Here's how the part is built. I have some questions about the finished solid (model axes, mm). A direction names the side the tool comes from. Round coordinates to 2 decimals unless told otherwise and drop trailing zeros. Loops run counter-clockwise (first coordinate to the right, second up) from the corner with the lowest first, then second, coordinate; pieces in that order, holes last. Notation, with made-up numbers: M 34,15 L 64,15 A19 ccw 64,33 Z; hole C 75,-32 d7. An arc over 180 degrees is marked long. Use a Markdown table: item, result.
from build123d import *

# Parameters (mm, degrees)
SKETCH2_W                = 3.0000000000000036
SKETCH2_H                = 3.9999999999999982
BOSS_EXTRUDE2_DEPTH      = 100
BOSS_EXTRUDE3_DEPTH      = 30
BOSS_EXTRUDE3_DEPTH_BACK = 105
FILLET5_R                = 10
FILLET6_R                = 5
FILLET7_R                = 2
FILLET8_R                = 1


with BuildPart() as part:
    # Sketch2 → Boss-Extrude2 (new body)
    with BuildSketch(Plane(origin=(0, 0, 0), x_dir=(0, 0, -1), z_dir=(1, 0, 0))):
        Polygon((8.660254037844407, 18.999999999999996), (24.660254037844407, 19), (27.660254037844407, 19), (27.660254037844407, 23), (8.660254037844407, 22.999999999999996), align=None)
        with Locations((26.160254037844403, 17)):
            Rectangle(SKETCH2_W, SKETCH2_H)
        Polygon((24.660254037844407, 15), (18.66025403784441, 15), (16.3508529610859, 10.999999999999996), (27.66025403784441, 11), (27.660254037844407, 15), align=None)
        Polygon((18.66025403784441, 15), (8.660254037844407, 15), (8.660254037844409, 11), (16.3508529610859, 11), align=None)
        with BuildLine():
            Line((8.660254037844407, 15.000000000000002), (0, 0))
            Line((0, 0), (3.2679491924311206, 1.4e-16))
            Line((3.2679491924311206, -8.2e-16), (6.165063509461155, 5.017949192431213))
            ThreePointArc((6.165063509461059, 5.017949192431232), (7.962900689456138, 8.449244298165432), (10.964101615137764, 6))
            ThreePointArc((10.964101615137764, 5.999999999999999), (10.334608934582356, 4.341325116876664), (8.763139720814397, 3.5179491924311193))
            Line((8.763139720814408, 3.5179491924311046), (6.732050807568877, 0))
            Line((6.732050807568877, 2.8e-16), (10.000000000000004, 4.1e-16))
            Line((10.000000000000004, -1.78e-15), (16.3508529610859, 10.999999999999996))
            Line((16.3508529610859, 11), (8.660254037844409, 11))
            Line((8.660254037844409, 11), (8.660254037844407, 15))
        make_face()
    extrude(amount=BOSS_EXTRUDE2_DEPTH)

    # Sketch3 → Boss-Extrude3 (add, two sides: drawn at the far end of the back side and taken through both)
    with BuildSketch(Plane(origin=(100, 0, 0), x_dir=(0, 0, -1), z_dir=(1, 0, 0)).offset(-BOSS_EXTRUDE3_DEPTH_BACK)):
        with BuildLine():
            Line((8.66025403784439, 15.000000000000005), (0, 0))
            Line((0, 0), (3.2679491924311215, 2.8e-16))
            Line((3.267949192431121, 0), (6.1650635094611035, 5.017949192431125))
            ThreePointArc((6.165063509461104, 5.017949192431125), (7.962900689456081, 8.449244298165421), (10.964101615137764, 6))
            ThreePointArc((10.964101615137764, 5.999999999999999), (10.334608934582363, 4.341325116876672), (8.763139720814419, 3.517949192431122))
            Line((8.763139720814419, 3.517949192431122), (6.732050807568878, 3.6e-16))
            Line((6.732050807568878, 3.6e-16), (10.000000000000002, 8.7e-16))
            Line((10.000000000000004, 0), (18.66025403784441, 15.000000000000009))
            Line((18.66025403784441, 15.000000000000009), (8.66025403784439, 15.000000000000005))
        make_face()
    extrude(amount=BOSS_EXTRUDE3_DEPTH + BOSS_EXTRUDE3_DEPTH_BACK)

    # Fillet5
    fillet5_edges = [part.edges().sort_by_distance(p)[0] for p in [
        (50, 10.999999999999998, -16.3508529610859),
    ]]
    fillet(fillet5_edges, radius=FILLET5_R)

    # Fillet6
    fillet6_edges = [part.edges().sort_by_distance(p)[0] for p in [
        (0, 10.500000000000007, -16.062177826491087),
        (100, 10.500000000000007, -16.062177826491087),
    ]]
    fillet(fillet6_edges, radius=FILLET6_R - 0.0001)  # a hair under: the kernel refuses the full size

    # Fillet7
    fillet7_edges = [part.edges().sort_by_distance(p)[0] for p in [
        (50, 23, -27.660254037844407),
        (50, 11, -27.66025403784441),
    ]]
    fillet(fillet7_edges, radius=FILLET7_R)

    # Fillet8
    fillet8_edges = [part.edges().sort_by_distance(p)[0] for p in [
        (62.5, 4.3e-16, -10.000000000000004),
        (62.5, 0, 0),
    ]]
    fillet(fillet8_edges, radius=FILLET8_R)


solid = part.part
1. I need wall thicknesses on probe 1 along Y at (x, z) = (2, -10.25); probe 2 along X at (y, z) = (12.5, -26); probe 3 along Y at (x, z) = (48, -16.5). Which ranges of each line are inside material? Lowest first, please. Write a range as from..to.
Answer sheet:
| item | result |
|---|---|
| probe 1 | 0.44..4.25, 7.75..15, 19..23 |
| probe 2 | 0..100 |
| probe 3 | 9.27..15, 19..23 |
2. Imagine slicing it at A-A, the plane x = 107. Write out the boundary of the cut face in (y, z).
Answer sheet:
| item | result |
|---|---|
| outline | M 0,-9.42 A1 ccw 0.5,-10.29 L 15,-18.66 L 15,-8.66 L 1.5,-0.87 A1 ccw 0,-1.73 L 0,-3.27 L 5.02,-6.17 A2.5 cw long 3.52,-8.76 L 0,-6.73 Z |
3. We'd pull the mould along Y, two halves only. Please class faces 5 (the face through (102.18, 12.67, -18.32)), 6 (the face through (49, 19, -17)), 7 (the face through (49, 21, -8.66)), 8 (the face through (62, 15, -17)): +Y half, -Y half, draft (parallel to the pull), parting line (faces both ways), or undercut.
Answer sheet:
| item | result |
|---|---|
| face 5 | -Y half |
| face 6 | undercut |
| face 7 | draft |
| face 8 | undercut |
4. Imagine slicing it at B-B, the plane x = 72. Write out the boundary of the cut face in (y, z), then the cut area to 3 significant figures.
Answer sheet:
| item | result |
|---|---|
| outline | M 0,-9.42 A1 ccw 0.5,-10.29 L 6,-13.46 A10 cw 11,-22.12 L 11,-25.66 A2 ccw 13,-27.66 L 21,-27.66 A2 ccw 23,-25.66 L 23,-8.66 L 19,-8.66 L 19,-24.66 L 15,-24.66 L 15,-8.66 L 1.5,-0.87 A1 ccw 0,-1.73 L 0,-3.27 L 5.02,-6.17 A2.5 cw long 3.52,-8.76 L 0,-6.73 Z |
| area | 248 mm2 |
5. Imagine slicing it at C-C, the plane y = 17.75. Write out the boundary of the cut face in (x, z), then the cut area to 3 significant figures.
Answer sheet:
| item | result |
|---|---|
| outline | M 0,-27.66 L 100,-27.66 L 100,-24.66 L 0,-24.66 Z |
| area | 300 mm2 |
6. For pin 1 Ø5 at (x, y) = (104, 20) entering from -Z; pin 2 Ø5 at (x, y) = (29.5, 8) entering from +Z; pin 3 Ø4 at (x, z) = (34.5, -24.5) entering from -Y; pin 4 Ø1 at (y, z) = (20, -15.5) entering from +X, each with a flat end and sliding along its axis, tell me the tip position at first contact or that it passes through.
Answer sheet:
| item | result |
|---|---|
| pin 1 | through |
| pin 2 | z = -3.18 |
| pin 3 | y = 11 |
| pin 4 | x = 100 |
7. Which directions (+Z, -Z, +X, -X, +Y, -Y) give clear straight access to the entire face, cutting with the end or side of a thin tool? Please do faces 1 (the face through (49, 11, -24)), 2 (the face through (61.55, 1.78, -7.76)), 3 (the face through (61.555, 2.474, -4.696)), 4 (the face through (76.555, 4.426, -12.556)).
Answer sheet:
| item | result |
|---|---|
| face 1 | -Z, +X, -X, -Y |
| face 2 | +X, -X |
| face 3 | +X, -X, -Y |
| face 4 | -Z, +X, -Y |
